Read the model definition and answer for the solid it produces. Units are mm, in the model's axes. Give positions to 0.01 mm unless a question says otherwise; leave off trailing zeros. Loops run counter-clockwise (first coordinate to the right, second up) from the corner with the lowest first, then second, coordinate; pieces in that order, holes last. Notation, with made-up numbers: (46, 33) -> (71, 33) arc R22 ccw to (71, 43) -> close; hole circle Ø8 at (86, 14.25). An arc over 180 degrees is marked (long way). Write each question's results on one line, items separated by ' | '. Start each with the question number.
Item 1: Section A-A on z = 0.9 is taken. Write down the section's boundary in (x, y) (3 decimals).
Item 2: Section B-B on x = -12 is taken. Write down the section's boundary in (y, z), and give its area (3 significant figures).
Item 3: Find the intervals of material crossed by line 1 (Y direction, x = -1.5, z = 2.7), in increasing order.
Item 4: Each of these flat-tipped pins is pushed along its axis until it touches: P1, Ø1.5, axis at y = -57, z = 2, coming from the -X side (3 decimals); P2, Ø0.9, axis at y = 57.5, z = 1, coming from the +X side (3 decimals); P3, Ø0.9, axis at x = -39, z = 2, coming from the -Y side. Where does it stop, or does it pass through?
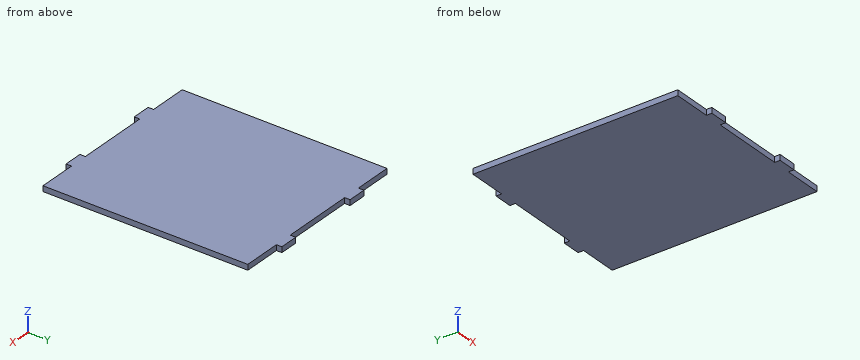
Autodesk Inventor part; units mm, degrees
ref_plane "Work Plane1" through (-19.935, -55, 0) normal (0, -1, 0) x (1, 0, 0)
ref_plane "YZ Plane" through (0, 0, 0) normal (1, 0, 0) x (0, 1, 0)
ref_plane "XZ Plane" through (0, 0, 0) normal (0, 1, 0) x (-1, 0, 0)
sketch "Sketch1" plane through (0, 0, 0) normal (0, 0, 1) x (1, 0, 0)
  line L0 (-51, 56) -> (51, 56)
  line L1 (51, 56) -> (51, -56)
  line L2 (51, -56) -> (-51, -56)
  line L3 (-51, -56) -> (-51, 56)
  line L4 (-51, 56) -> (51, -56) construction
  line L5 (51, 56) -> (-51, -56) construction
  point P0 (0, 0)
  point P1 (0, 0)
  point P2 (0, 0)
  dimension "d0" = 102
  dimension "d1" = 112
extrude "Extrusion1" add sketch "Sketch1" along normal blind 3
sketch "Sketch2" plane through (0, 0, 3) normal (0, 0, 1) x (1, 0, 0)
  line L0 (-51, -56) -> (51, -56)
  line L1 (-30.065, -59) -> (-19.935, -59)
  line L2 (-19.935, -59) -> (-19.935, -56)
  line L3 (-19.935, -56) -> (-30.065, -56)
  line L4 (-30.065, -56) -> (-30.065, -59)
  line L5 (-30.065, -59) -> (-19.935, -56) construction
  line L6 (-19.935, -59) -> (-30.065, -56) construction
  line L7 (19.935, -59) -> (30.065, -59)
  line L8 (30.065, -59) -> (30.065, -56)
  line L9 (30.065, -56) -> (19.935, -56)
  line L10 (19.935, -56) -> (19.935, -59)
  line L11 (19.935, -59) -> (30.065, -56) construction
  line L12 (30.065, -59) -> (19.935, -56) construction
  point P0 (0, 0)
  point P1 (-25, -57.5)
  point P2 (25, -57.5)
  dimension "d4" = 3
  dimension "d5" = 25
  dimension "d6" = 25
  dimension "d7" = 10.13
  dimension "d8" = 10.13
extrude "Extrusion2" add sketch "Sketch2" against normal blind 3
mirror "Mirror1" about plane through (0, 0, 0) normal (0, 1, 0) of "Extrusion2"
sketch "Sketch3" plane through (0, 0, 0) normal (0, 0, -1) x (-1, 0, 0)
  line L0 (-51, -56) -> (-51, 56) construction
  line L1 (-51, 55) -> (51, 55) construction
  line L2 (51, 56) -> (51, -56) construction
  line L3 (-51, -55) -> (51, -55) construction
  line L4 (-19.935, -56) -> (19.935, -56) construction
  line L5 (-30.065, 56) -> (-51, 56) construction
  point P0 (0, 0)
  dimension "d11" = 1
  dimension "d12" = 1
ref_plane "Work Plane1" through (-19.935, -55, 0) normal (0, -1, 0) x (1, 0, 0)
sketch "Sketch6" plane through (0, 0, 3) normal (0, 0, 1) x (1, 0, 0)
  line L0 (30.065, -56) -> (51, -56)
  line L1 (51, -56) -> (51, 56)
  point P0 (0, 0)
  point P1 (20.6, -36.4)
  dimension "d41" = 19.6
  dimension "d42" = 30.4
hole "Hole4" [suppressed]
pattern_linear "Rectangular Pattern1" [suppressed]
sketch "Sketch7" plane through (0, 0, 3) normal (0, 0, 1) x (1, 0, 0)
  spline S0 degree 3 poles (-17.7549, 22.0592) (-20.3586, 22.7486) (-27.8891, 27.7258) (-21.8129, 49.2984) knots 3 3 3 3 4 4 4 4
  line L0 (-20.3586, 22.7486) -> (-27.8891, 27.7258) construction
  line L1 (-17.7549, 22.0592) -> (-20.3586, 22.7486) construction
  line L2 (-27.8891, 27.7258) -> (-21.8129, 49.2984) construction
  spline S1 degree 3 poles (-35.4301, 25.2372) (-34.47, 24.8476) (-28.6027, 22.0592) (-17.7549, 22.0592) knots 2 2 2 2 3 3 3 3
  line L3 (-35.4301, 25.2372) -> (-34.47, 24.8476) construction
  line L4 (-34.47, 24.8476) -> (-28.6027, 22.0592) construction
  line L5 (-28.6027, 22.0592) -> (-17.7549, 22.0592) construction
  spline S2 degree 3 poles (-41.3451, 44.549) (-42.3928, 42.443) (-47.2601, 32.6596) (-35.4301, 25.2372) knots 1 1 1 1 2 2 2 2
  line L6 (-41.3451, 44.549) -> (-42.3928, 42.443) construction
  line L7 (-42.3928, 42.443) -> (-47.2601, 32.6596) construction
  line L8 (-47.2601, 32.6596) -> (-35.4301, 25.2372) construction
  spline S3 degree 3 poles (-37.458, 43.3832) (-40.0894, 43.0815) (-41.2381, 43.3832) (-41.3451, 44.549) knots 0 0 0 0 1 1 1 1
  line L9 (-40.0894, 43.0815) -> (-41.2381, 43.3832) construction
  line L10 (-37.458, 43.3832) -> (-40.0894, 43.0815) construction
  line L11 (-41.2381, 43.3832) -> (-41.3451, 44.549) construction
  spline S4 degree 3 poles (-21.8129, 49.2984) (-21.8202, 49.2933) (-29.1299, 44.232) (-37.458, 43.3832) knots 4 4 4 4 5 5 5 5
  line L12 (-21.8129, 49.2984) -> (-29.1299, 44.232) construction
  line L13 (-29.1299, 44.232) -> (-37.458, 43.3832) construction
  spline S5 degree 3 poles (-15.7483, 21.8123) (-16.0581, 21.8979) (-29.0611, 22.4788) (-21.0119, 50.2568) knots 3 3 3 3 4 4 4 4
  line L14 (-15.7483, 21.8123) -> (-16.0581, 21.8979) construction
  line L15 (-16.0581, 21.8979) -> (-29.0611, 22.4788) construction
  line L16 (-29.0611, 22.4788) -> (-21.0119, 50.2568) construction
  spline S6 degree 3 poles (-21.0119, 50.2568) (-21.2194, 50.1207) (-29.151, 44.9225) (-36.6832, 43.8886) knots 4 4 4 4 5 5 5 5
  line L17 (-21.0119, 50.2568) -> (-21.2194, 50.1207) construction
  line L18 (-21.2194, 50.1207) -> (-29.151, 44.9225) construction
  line L19 (-29.151, 44.9225) -> (-36.6832, 43.8886) construction
  line L20 (-36.6832, 43.8886) -> (-35.9502, 47.0532)
  spline S7 degree 3 poles (-35.9502, 47.0532) (-35.9625, 47.0497) (-40.7954, 45.8307) (-41.6808, 44.7755) knots 0 0 0 0 1 1 1 1
  line L21 (-35.9502, 47.0532) -> (-35.9625, 47.0497) construction
  line L22 (-35.9625, 47.0497) -> (-40.7954, 45.8307) construction
  line L23 (-40.7954, 45.8307) -> (-41.6808, 44.7755) construction
  spline S8 degree 3 poles (-41.6808, 44.7755) (-41.6808, 44.7755) (-49.0375, 32.8716) (-35.5714, 24.8043) knots 1 1 1 1 2 2 2 2
  line L24 (-41.6808, 44.7755) -> (-41.6808, 44.7755) construction
  line L25 (-41.6808, 44.7755) -> (-49.0375, 32.8716) construction
  line L26 (-49.0375, 32.8716) -> (-35.5714, 24.8043) construction
  spline S9 degree 3 poles (-35.5714, 24.8043) (-35.5511, 24.7921) (-28.5456, 20.8762) (-15.7483, 21.8123) knots 2 2 2 2 3 3 3 3
  line L27 (-35.5714, 24.8043) -> (-35.5511, 24.7921) construction
  line L28 (-35.5511, 24.7921) -> (-28.5456, 20.8762) construction
  line L29 (-28.5456, 20.8762) -> (-15.7483, 21.8123) construction
  line L30 (-15.2682, 33.8195) -> (-22.3387, 33.8195) construction
  line L31 (-22.3387, 33.8195) -> (-22.3387, 39.2773) construction
  line L32 (-22.3387, 39.2773) -> (-15.2682, 39.2773) construction
  line L33 (-15.2682, 39.2773) -> (-15.2682, 33.8195) construction
  line L34 (-24.7016, 33.8748) -> (-43.5687, 33.8748) construction
  line L35 (-43.5687, 33.8748) -> (-43.5687, 39.6523) construction
  line L36 (-43.5687, 39.6523) -> (-24.7016, 39.6523) construction
  line L37 (-24.7016, 39.6523) -> (-24.7016, 33.8748) construction
  line L38 (-13.4408, 37.5513) -> (-45.6182, 37.5513) construction
  spline S10 degree 3 poles (38.6981, -46.4393) (32.5457, -44.8102) (14.7509, -33.0491) (29.1091, 17.9269) knots 3 3 3 3 4 4 4 4
  line L39 (38.6981, -46.4393) -> (32.5457, -44.8102) construction
  line L40 (32.5457, -44.8102) -> (14.7509, -33.0491) construction
  line L41 (14.7509, -33.0491) -> (29.1091, 17.9269) construction
  spline S11 degree 3 poles (-3.0683, -38.9296) (-0.7996, -39.8503) (13.0647, -46.4393) (38.6981, -46.4393) knots 2 2 2 2 3 3 3 3
  line L42 (-3.0683, -38.9296) -> (-0.7996, -39.8503) construction
  line L43 (-0.7996, -39.8503) -> (13.0647, -46.4393) construction
  line L44 (13.0647, -46.4393) -> (38.6981, -46.4393) construction
  spline S12 degree 3 poles (-17.0455, 6.7041) (-19.5213, 1.7277) (-31.0226, -21.3906) (-3.0683, -38.9296) knots 1 1 1 1 2 2 2 2
  line L45 (-17.0455, 6.7041) -> (-19.5213, 1.7277) construction
  line L46 (-19.5213, 1.7277) -> (-31.0226, -21.3906) construction
  line L47 (-31.0226, -21.3906) -> (-3.0683, -38.9296) construction
  spline S13 degree 3 poles (-7.8603, 3.9492) (-14.0782, 3.2364) (-16.7927, 3.9492) (-17.0455, 6.7041) knots 0 0 0 0 1 1 1 1
  line L48 (-7.8603, 3.9492) -> (-14.0782, 3.2364) construction
  line L49 (-14.0782, 3.2364) -> (-16.7927, 3.9492) construction
  line L50 (-16.7927, 3.9492) -> (-17.0455, 6.7041) construction
  spline S14 degree 3 poles (29.1091, 17.9269) (29.0918, 17.9149) (11.819, 5.9549) (-7.8603, 3.9492) knots 4 4 4 4 5 5 5 5
  line L51 (29.1091, 17.9269) -> (11.819, 5.9549) construction
  line L52 (11.819, 5.9549) -> (-7.8603, 3.9492) construction
  spline S15 degree 3 poles (43.4399, -47.0227) (42.7078, -46.8204) (11.9815, -45.4479) (31.0019, 20.1915) knots 3 3 3 3 4 4 4 4
  line L53 (43.4399, -47.0227) -> (42.7078, -46.8204) construction
  line L54 (42.7078, -46.8204) -> (11.9815, -45.4479) construction
  line L55 (11.9815, -45.4479) -> (31.0019, 20.1915) construction
  spline S16 degree 3 poles (31.0019, 20.1915) (30.5115, 19.8701) (11.7692, 7.5867) (-6.0293, 5.1437) knots 4 4 4 4 5 5 5 5
  line L56 (31.0019, 20.1915) -> (30.5115, 19.8701) construction
  line L57 (30.5115, 19.8701) -> (11.7692, 7.5867) construction
  line L58 (11.7692, 7.5867) -> (-6.0293, 5.1437) construction
  line L59 (-6.0293, 5.1437) -> (-4.2974, 12.6214)
  spline S17 degree 3 poles (-4.2974, 12.6214) (-4.3264, 12.6132) (-15.7465, 9.7327) (-17.8388, 7.2392) knots 0 0 0 0 1 1 1 1
  line L60 (-4.2974, 12.6214) -> (-4.3264, 12.6132) construction
  line L61 (-4.3264, 12.6132) -> (-15.7465, 9.7327) construction
  line L62 (-15.7465, 9.7327) -> (-17.8388, 7.2392) construction
  spline S18 degree 3 poles (-17.8388, 7.2392) (-17.8388, 7.2392) (-35.2226, -20.8896) (-3.4022, -39.9527) knots 1 1 1 1 2 2 2 2
  line L63 (-17.8388, 7.2392) -> (-17.8388, 7.2392) construction
  line L64 (-17.8388, 7.2392) -> (-35.2226, -20.8896) construction
  line L65 (-35.2226, -20.8896) -> (-3.4022, -39.9527) construction
  spline S19 degree 3 poles (-3.4022, -39.9527) (-3.3542, -39.9815) (13.1998, -49.2348) (43.4399, -47.0227) knots 2 2 2 2 3 3 3 3
  line L66 (-3.4022, -39.9527) -> (-3.3542, -39.9815) construction
  line L67 (-3.3542, -39.9815) -> (13.1998, -49.2348) construction
  line L68 (13.1998, -49.2348) -> (43.4399, -47.0227) construction
  line L69 (44.5744, -18.6497) -> (27.8666, -18.6497) construction
  line L70 (27.8666, -18.6497) -> (27.8666, -5.753) construction
  line L71 (27.8666, -5.753) -> (44.5744, -5.753) construction
  line L72 (44.5744, -5.753) -> (44.5744, -18.6497) construction
  line L73 (22.2831, -18.519) -> (-22.2999, -18.519) construction
  line L74 (-22.2999, -18.519) -> (-22.2999, -4.8668) construction
  line L75 (-22.2999, -4.8668) -> (22.2831, -4.8668) construction
  line L76 (22.2831, -4.8668) -> (22.2831, -18.519) construction
  line L77 (48.8924, -17.3822) -> (-27.1429, -9.8315) construction
  point P0 (0, 0)
  point P1 (-46.1734, 35.5024)
  point P2 (-28.4547, -14.6731)
  point P3 (36.4717, -44.6082)
  point P4 (32.5457, -41.4669)
  point P5 (29.1091, -36.761)
  point P6 (27.1695, -32.4025)
  point P7 (25.7734, -27.2321)
  point P8 (24.9854, -21.3562)
  point P9 (24.7959, -14.6712)
  point P10 (25.3026, -6.9857)
  point P11 (26.1472, -0.3981)
  point P12 (27.414, 5.5982)
  point P13 (28.9178, 11.9055)
  point P14 (23.0904, 15.6216)
  point P15 (16.165, 12.2433)
  point P16 (8.2261, 8.9495)
  point P17 (0.7095, 6.6692)
  point P18 (-13.648, 9.5407)
  point P19 (-20.2241, 2.0414)
  point P20 (-22.4199, -6.8265)
  point P21 (-21.9132, -16.5389)
  point P22 (-18.6194, -25.4913)
  point P23 (-13.721, -31.9099)
  point P24 (-8.4465, -36.7937)
  point P25 (-1.1832, -41.0165)
  point P26 (7.0934, -43.888)
  point P27 (14.1878, -45.4927)
  point P28 (21.8732, -46.6751)
  point P29 (34.6261, -47.3507)
  point P30 (28.2919, -47.1818)
  point P31 (-5.2552, 8.4859)
  point P32 (-13.2219, 3.7788)
  point P33 (-8.6285, 11.4147)
  point P34 (-16.5626, 5.2105)
  point P35 (-9.2199, 3.595)
hole "Hole5" [suppressed]
equation "\"d8\" = d7"
equation "\"d12\" = d11"
equation "\"kerf\" = 0.13"
properties part number "TopPanel" material "Acrylic, Clear"
Findings:
1) outline: (-51, -56) -> (-30.065, -56) -> (-30.065, -59) -> (-19.935, -59) -> (-19.935, -56) -> (19.935, -56) -> (19.935, -59) -> (30.065, -59) -> (30.065, -56) -> (51, -56) -> (51, 56) -> (30.065, 56) -> (30.065, 59) -> (19.935, 59) -> (19.935, 56) -> (-19.935, 56) -> (-19.935, 59) -> (-30.065, 59) -> (-30.065, 56) -> (-51, 56) -> close
2) outline: (-56, 0) -> (56, 0) -> (56, 3) -> (-56, 3) -> close | area: 336 mm2
3) line 1: -56 to 56
4) P1: x = -30.065 | P2: x = 30.065 | P3: y = -56
